```python
from build123d import *

# Parameters (mm, degrees)
SKETCH_2_W                   = 78
SKETCH_2_H                   = 40
EXTRUDE_1_DEPTH              = 2
SKETCH_3_R                   = 5.05
SKETCH_3_R_2                 = 1.25
CUT_EXTRUDE_1_DEPTH          = 88.681240867
SKETCH_4_R                   = 1.25
CUT_EXTRUDE_2_DEPTH          = 88.681240867
FILLET_1_R                   = 20
HOLE_WIZARD_M3_1_D           = 2.5
HOLE_WIZARD_M3_1_CSINK_D     = 2.55
HOLE_WIZARD_M3_1_CSINK_ANGLE = 90


with BuildPart() as part:
    # 草图2 → 凸台-拉伸1 (new body)
    with BuildSketch(Plane.XY):
        with Locations((39, 20)):
            Rectangle(SKETCH_2_W, SKETCH_2_H)
    extrude(amount=EXTRUDE_1_DEPTH)

    # 草图3 → 切除-拉伸1 (cut, through all)
    with BuildSketch(Plane(origin=(0, 0, 0), x_dir=(-1, 0, 0), z_dir=(0, 0, -1))):
        with Locations((-20, 20)):
            Circle(SKETCH_3_R)
        with Locations((-10, 10.202041029)):
            Circle(SKETCH_3_R_2)
        with BuildLine():
            ThreePointArc((-30.446428571, 32.447274003), (-34.413244876, 12.495276677), (-15.792765742, 4.30408716))
            ThreePointArc((-15.792765742, 4.30408716), (-14.20202563, 7.059907527), (-16.957845998, 8.650647638))
            ThreePointArc((-16.957845998, 8.650647638), (-30.421884756, 14.573507751), (-27.553571429, 29.000336587))
            ThreePointArc((-27.553571429, 29.000336587), (-27.276531292, 32.170233866), (-30.446428571, 32.447274003))
        make_face()
    extrude(amount=-CUT_EXTRUDE_1_DEPTH, mode=Mode.SUBTRACT)

    # 草图4 → 切除-拉伸2 (cut, through all)
    with BuildSketch(Plane(origin=(0, 0, 0), x_dir=(-1, 0, 0), z_dir=(0, 0, -1))):
        with Locations((-73, 34)):
            Circle(SKETCH_4_R)
        with Locations((-73, 10)):
            Circle(SKETCH_4_R)
    extrude(amount=-CUT_EXTRUDE_2_DEPTH, mode=Mode.SUBTRACT)

    # 圆角1
    fillet_1_edges = [part.edges().sort_by_distance(p)[0] for p in [
        (0, 40, 1),
        (0, 0, 1),
    ]]
    fillet(fillet_1_edges, radius=FILLET_1_R - 0.0001)  # a hair under: the kernel refuses the full size

    # M3 螺纹孔的螺纹孔钻头1 (through all)
    with Locations(Plane(origin=(73, 34, 0), x_dir=(-1, 0, 0), z_dir=(0, 0, -1))):
        with Locations((0, 0), (0, -24)):
            CounterSinkHole(HOLE_WIZARD_M3_1_D / 2, HOLE_WIZARD_M3_1_CSINK_D / 2, counter_sink_angle=HOLE_WIZARD_M3_1_CSINK_ANGLE)


solid = part.part
```
Can you work these out from the model? Positions are in its coordinate system, mm. Round coordinates to 2 decimals unless told otherwise and drop trailing zeros. Order: outer loops, then holes, each group sorted by start corner. A loop starts at its lowest first (then second) coordinate and runs counter-clockwise, first axis right, second up. Notation, with made-up numbers: (8.25, 67.25) -> (31.25, 67.25) arc R18 cw to (31.25, 87.25) -> close; hole circle Ø11 at (70, 69). An arc over 180 degrees is marked (long way). Return JSON: item names as keys, results as strings. Group by question number.
1. Will these pins go through, and if not, where does the flat tip stop? pin 1 (1 mm diameter, centred on y = 27, z = 2, fed in from -X); pin 2 (1.5 mm diameter, centred on x = 73, y = 34, fed in from -Z).
2. I need wall thicknesses on line 1 (Y direction, x = 73, z = 1); line 2 (X direction, y = 19, z = 1.75); line 3 (X direction, y = 24.5, z = 1.4). Which ranges of each line are inside material? Lowest first, please. Write a range as [from, to].
3. If we section it at B-B, the plane z = 1.1: Count the separate pieces of the cut face and the enclosed holes in it, then the cut area to 3 significant figures.
4. If we section it at A-A, the plane y = 34: Write out the boundary of the cut face in (x, z) (3 decimals), then the cut area to 3 significant figures.
5. If we section it at C-C, the plane x = 29: Write out the boundary of the cut face in (y, z).
6. We'd pull the mould along X, two halves only. Please class faces 1 (the face through (27.245, 32.132, 0.986)), 2 (the face through (49, 40, 1)), 3 (the face through (5.703, 33.986, 1.014)): released by +X, released by -X, zero draft, split by the parting line, or undercut.
Output values:
{
 "1": {"pin 1": "x = 1.09", "pin 2": "through"},
 "2": {"line 1": "[0, 8.75], [11.25, 32.75], [35.25, 40]", "line 2": "[0.03, 15.05], [24.95, 31.71], [36.22, 78]", "line 3": "[0.51, 17.71], [22.29, 30.85], [35.61, 78]"},
 "3": {"separate pieces": "1", "enclosed holes": "5", "area": "2,670 mm²"},
 "4": {"outline": "(5.717, 0) -> (71.725, 0) -> (71.75, 0.025) -> (71.75, 2) -> (5.717, 2) -> close; (74.25, 0.025) -> (74.275, 0) -> (78, 0) -> (78, 2) -> (74.25, 2) -> close", "area": "140 mm²"},
 "5": {"outline": "(0, 0) -> (6.47, 0) -> (6.47, 2) -> (0, 2) -> close; (12.45, 0) -> (27.55, 0) -> (27.55, 2) -> (12.45, 2) -> close; (32.97, 0) -> (40, 0) -> (40, 2) -> (32.97, 2) -> close"},
 "6": {"face 1": "undercut", "face 2": "zero draft", "face 3": "released by -X"}
}
